Could you check a few things on this model? Use its own coordinates, in mm. A direction names the side the tool comes from. Coordinates: 2 decimals unless noted, no trailing zeros. Write each loop counter-clockwise with the first axis right and the second up, starting at its lowest first coordinate (ties: lowest second). Pieces come first, ordered by that corner, then holes. Notation, with made-up numbers: (5.5, 67) - (63.5, 67) arc R26 cw to (63.5, 95) - close; hole circle Ø4 at (88.25, 88). An arc over 180 degrees is marked (long way). Write item = value, one per line. Start each with the question number.
```python
from build123d import *

# Parameters (mm, degrees)
F0_R     = 2.5
F0_R_2   = 1.5
F1_DEPTH = 4
F0_R_3   = 5
F2_DEPTH = 1
F3_R     = 5
F3_R_2   = 2.5
F3_R_3   = 1.5
F4_DEPTH = 1


with BuildPart() as f1:
    # F0 (on Top) → F1 (new body)
    with BuildSketch(Plane.XY):
        Circle(F0_R)
        Circle(F0_R_2, mode=Mode.SUBTRACT)
    extrude(amount=F1_DEPTH)

    # F0 (on Top) → F2 (join)
    with BuildSketch(Plane.XY):
        Circle(F0_R_3)
        Circle(F0_R, mode=Mode.SUBTRACT)
    extrude(amount=F2_DEPTH)

    # F3 (on face) → F4 (join)
    with BuildSketch(Plane.XY.offset(4)):
        Circle(F3_R)
        Circle(F3_R_2, mode=Mode.SUBTRACT)
        Circle(F3_R_2)
        Circle(F3_R_3, mode=Mode.SUBTRACT)
    extrude(amount=-F4_DEPTH)


solid = f1.part
```
1) Which directions (+Z, -Z, +X, -X, +Y, -Y) give clear straight access to the entire face, cutting with the end or side of a thin tool? Please do faces 5 (the cylindrical face through (-1.5, 0.07, 1.97)), 6 (the cylindrical face through (-0.54, -2.44, 1.99)).
2) Suppose I cut it at B-B on y = 3.5. Please give me the cut outline in (x, z).
3) Thinking about a two-plate mould opening in Z: for faces 1 (the flat face through (2, -2, 1)), 2 (the flat face through (-1.2, 1.2, 0)), 3 (the cylindrical face through (-1.08, -4.88, 0.49)), 4 (the flat face through (-1.2, 1.2, 4)), which applies, +Z half, -Z half, draft (parallel to the pull), parting line (faces both ways), or undercut?
4) For P1, Ø1, axis at y = 1.5, z = 0.5, coming from the +X side; P2, Ø1.5, axis at y = 3, z = 1.5, coming from the -X side, each with a flat end and sliding along its axis, tell me the tip position at first contact or that it passes through.
5) Suppose I cut it at D-D on y = 2.25. Please give me the cut outline in (x, z).
6) Suppose I cut it at A-A on x = 0. Please give me the cut outline in (y, z), plus the area to 3 significant figures.
7) Suppose I cut it at C-C on z = 1.35. Please give me the cut outline in (x, y), plus the area to 3 significant figures.
8) If I drill on probe 1 along Y at (x, z) = (0, 1.85); probe 2 along Z at (x, y) = (4, -0.25); probe 3 along X at (y, z) = (0.75, 2.65), over which ranges is the centre line in solid material (lowest first)? Write a range as [from, to].
Reply:
q1.face_5 = +Z, -Z
q1.face_6 = none
q2.outline = (-3.57, 0) - (3.57, 0) - (3.57, 1) - (-3.57, 1) - close; (-3.57, 3) - (3.57, 3) - (3.57, 4) - (-3.57, 4) - close
q3.face_1 = undercut
q3.face_2 = -Z half
q3.face_3 = draft
q3.face_4 = +Z half
q4.P1 = 4.9
q4.P2 = -4.36
q5.outline = (-4.47, 0) - (4.47, 0) - (4.47, 1) - (1.09, 1) - (1.09, 3) - (4.47, 3) - (4.47, 4) - (-4.47, 4) - (-4.47, 3) - (-1.09, 3) - (-1.09, 1) - (-4.47, 1) - close
q6.outline = (-5, 0) - (-1.5, 0) - (-1.5, 4) - (-5, 4) - (-5, 3) - (-2.5, 3) - (-2.5, 1) - (-5, 1) - close; (1.5, 0) - (5, 0) - (5, 1) - (2.5, 1) - (2.5, 3) - (5, 3) - (5, 4) - (1.5, 4) - close
q6.area = 18.0 mm^2
q7.outline = circle Ø5 at (0, 0); hole circle Ø3 at (0, 0)
q7.area = 12.6 mm^2
q8.probe_1 = [-2.5, -1.5], [1.5, 2.5]
q8.probe_2 = [0, 1], [3, 4]
q8.probe_3 = [-2.38, -1.3], [1.3, 2.38]
